Geometry: final body of the model. Coordinates: model frame, mm. Give positions to 0.01 mm unless a question says otherwise; leave off trailing zeros. Order: outer loops, then holes, each group sorted by start corner. A loop starts at its lowest first (then second) coordinate and runs counter-clockwise, first axis right, second up. Notation, with made-up numbers: M 73.25,36 L 126.25,36 A20 cw 126.25,48 Z; hole C -30.75,88.5 d4. An arc over 180 degrees is marked long. One line per item, written item: value. Start each with the question number.
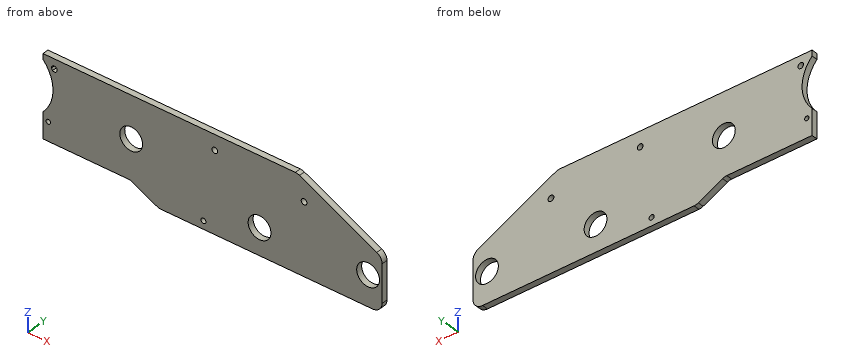
```python
from build123d import *

# Parameters (mm, degrees)
SKETCH1_W           = 210
SKETCH1_H           = 50
SKETCH1_R           = 1.211665018
SKETCH1_R_2         = 1.165617118
SKETCH1_R_3         = 1.5
SKETCH1_R_4         = 1.517273905
SKETCH1_R_5         = 1.335614121
SKETCH1_R_6         = 1.62438417
BOSS_EXTRUDE1_DEPTH = 3.175
SKETCH2_R           = 2
CUT_EXTRUDE1_DEPTH  = 10
SKETCH3_R           = 6
SKETCH3_R_2         = 0.586995366
CUT_EXTRUDE2_DEPTH  = 57.15
CUT_EXTRUDE7_DEPTH  = 10
FILLET3_R           = 5
SKETCH11_R          = 18.5
SKETCH11_R_2        = 2
BOSS_EXTRUDE4_DEPTH = 3.175
SKETCH12_R          = 21
BOSS_EXTRUDE5_DEPTH = 3.175
SKETCH13_R          = 18.85
CUT_EXTRUDE8_DEPTH  = 3.175
BOSS_EXTRUDE6_DEPTH = 3.175
FILLET4_R           = 5
SKETCH15_R          = 1.5
CUT_EXTRUDE9_DEPTH  = 10
SKETCH16_R          = 1.5
CUT_EXTRUDE10_DEPTH = 10
SKETCH17_R          = 1.5
CUT_EXTRUDE11_DEPTH = 10
CUT_EXTRUDE12_DEPTH = 10


with BuildPart() as part:
    # Sketch1 → Boss-Extrude1 (new body)
    with BuildSketch(Plane(origin=(0, 0, 0), x_dir=(1, 0, 0), z_dir=(0, 1, 0))):
        with Locations((105, -25)):
            Rectangle(SKETCH1_W, SKETCH1_H)
        with Locations(Location((3.489526233, -16.787661112, 0), (0, 0, 270))):
            Circle(SKETCH1_R, mode=Mode.SUBTRACT)
        with Locations(Location((34.37258772, -17.194005245, 0), (0, 0, 270))):
            Circle(SKETCH1_R_2, mode=Mode.SUBTRACT)
        with Locations(Location((37.520749958, -44.921198121, 0), (0, 0, 270))):
            Circle(SKETCH1_R_3, mode=Mode.SUBTRACT)
        with Locations(Location((168.975233936, -37.403209633, 0), (0, 0, 270))):
            Circle(SKETCH1_R_4, mode=Mode.SUBTRACT)
        with Locations(Location((116, -4.237214774, 0), (0, 0, 270))):
            Circle(SKETCH1_R_5, mode=Mode.SUBTRACT)
        with Locations(Location((12.257640281, -3.274812063, 0), (0, 0, 270))):
            Circle(SKETCH1_R_6, mode=Mode.SUBTRACT)
    extrude(amount=BOSS_EXTRUDE1_DEPTH)

    # Sketch2 → Cut-Extrude1 (cut)
    with BuildSketch(Plane(origin=(0, 3.175, 0), x_dir=(1, 0, 0), z_dir=(0, 1, 0))):
        with Locations(Location((10, -26, 0), (0, 0, 270))):
            Circle(SKETCH2_R)
        with Locations(Location((10, -42, 0), (0, 0, 270))):
            Circle(SKETCH2_R)
        with Locations(Location((26, -26, 0), (0, 0, 270))):
            Circle(SKETCH2_R)
        with Locations(Location((26, -42, 0), (0, 0, 270))):
            Circle(SKETCH2_R)
    extrude(amount=-CUT_EXTRUDE1_DEPTH, mode=Mode.SUBTRACT)

    # Sketch3 → Cut-Extrude2 (cut)
    with BuildSketch(Plane(origin=(0, 3.175, 0), x_dir=(1, 0, 0), z_dir=(0, 1, 0))):
        with Locations(Location((78.01026379, -28.1, 0), (0, 0, 270))):
            Circle(SKETCH3_R)
        with Locations(Location((145.531297368, -14, 0), (0, 0, 270))):
            Circle(SKETCH3_R)
        with Locations(Location((18, -34, 0), (0, 0, 270))):
            Circle(SKETCH3_R_2)
        with Locations(Location((202.646291021, -16, 0), (0, 0, 270))):
            Circle(SKETCH3_R)
    extrude(amount=-CUT_EXTRUDE2_DEPTH, mode=Mode.SUBTRACT)

    # Sketch10 → Cut-Extrude7 (cut)
    with BuildSketch(Plane(origin=(0, 3.175, 0), x_dir=(1, 0, 0), z_dir=(0, 1, 0))):
        Polygon((210, -27.859435908), (165.502877994, -50), (210, -50), align=None)
        Polygon((92.532613397, 0), (77.65477062, -7.402812063), (0, -7.402812063), (0, 0), align=None)
    extrude(amount=-CUT_EXTRUDE7_DEPTH, mode=Mode.SUBTRACT)

    # Fillet3
    fillet3_edges = [part.edges().sort_by_distance(p)[0] for p in [
        (210, 1.5875, 0),
        (0, 1.5875, 50),
        (92.532613397, 1.5875, 0),
        (210, 1.5875, 27.859435908),
        (165.502877994, 1.5875, 50),
        (77.65477062, 1.5875, 7.402812063),
        (0, 1.5875, 7.402812063),
    ]]
    fillet(fillet3_edges, radius=FILLET3_R)

    # Sketch11 → Boss-Extrude4 (add)
    with BuildSketch(Plane(origin=(0, 3.175, 0), x_dir=(1, 0, 0), z_dir=(0, 1, 0))):
        with Locations((18, -34)):
            Circle(SKETCH11_R)
        with Locations(Location((10, -26, 0), (0, 0, 270))):
            Circle(SKETCH11_R_2, mode=Mode.SUBTRACT)
        with Locations(Location((10, -42, 0), (0, 0, 270))):
            Circle(SKETCH11_R_2, mode=Mode.SUBTRACT)
        with Locations(Location((26, -26, 0), (0, 0, 270))):
            Circle(SKETCH11_R_2, mode=Mode.SUBTRACT)
        with Locations(Location((26, -42, 0), (0, 0, 270))):
            Circle(SKETCH11_R_2, mode=Mode.SUBTRACT)
    extrude(amount=-BOSS_EXTRUDE4_DEPTH)

    # Sketch12 → Boss-Extrude5 (add)
    with BuildSketch(Plane(origin=(0, 3.175, 0), x_dir=(1, 0, 0), z_dir=(0, 1, 0))):
        with Locations((18, -34)):
            Circle(SKETCH12_R)
    extrude(amount=-BOSS_EXTRUDE5_DEPTH)

    # Sketch13 → Cut-Extrude8 (cut)
    with BuildSketch(Plane(origin=(0, 3.175, 0), x_dir=(1, 0, 0), z_dir=(0, 1, 0))):
        with Locations(Location((18, -34, 0), (0, 0, 270))):
            Circle(SKETCH13_R)
    extrude(amount=-CUT_EXTRUDE8_DEPTH, mode=Mode.SUBTRACT)

    # Sketch14 → Boss-Extrude6 (add)
    with BuildSketch(Plane(origin=(0, 3.175, 0), x_dir=(1, 0, 0), z_dir=(0, 1, 0))):
        with BuildLine():
            Line((-35.83, -34.272812063), (-2.998227868, -34.272812063))
            ThreePointArc((-2.998227868, -34.272812063), (-2.272136238, -28.519079241), (0, -23.183346174))
            Line((0, -23.183346174), (0, -12.402812063))
            Line((0, -12.402812063), (0, -12.248529085))
            Line((0, -12.248529085), (0, 0.727187937))
            Line((0, 0.727187937), (-35.83, 0.727187937))
            Line((-35.83, 0.727187937), (-35.83, -34.272812063))
        make_face()
        with BuildLine():
            Line((0, 0.727187937), (0, -12.248529085))
            Line((0, -12.248529085), (0.002380891, -12.248529085))
            ThreePointArc((0.002380891, -12.248529085), (1.51944077, -8.813145304), (5, -7.402812063))
            Line((5, -7.402812063), (18, -7.402812063))
            Line((18, -7.402812063), (18, 0.727187937))
            Line((18, 0.727187937), (0, 0.727187937))
        make_face()
    extrude(amount=-BOSS_EXTRUDE6_DEPTH)

    # Fillet4
    fillet4_edges = [part.edges().sort_by_distance(p)[0] for p in [
        (-35.83, 1.5875, 34.272812063),
        (-35.83, 1.5875, -0.727187937),
        (18, 1.5875, -0.727187937),
    ]]
    fillet(fillet4_edges, radius=FILLET4_R)

    # Sketch15 → Cut-Extrude9 (cut)
    with BuildSketch(Plane(origin=(0, 3.175, 0), x_dir=(1, 0, 0), z_dir=(0, 1, 0))):
        with Locations(Location((122, -42.058139805, 0), (0, 0, 270))):
            Circle(SKETCH15_R)
    extrude(amount=-CUT_EXTRUDE9_DEPTH, mode=Mode.SUBTRACT)

    # Sketch16 → Cut-Extrude10 (cut)
    with BuildSketch(Plane(origin=(0, 3.175, 0), x_dir=(1, 0, 0), z_dir=(0, 1, 0))):
        with Locations(Location((12, -3.272812063, 0), (0, 0, 270))):
            Circle(SKETCH16_R)
    extrude(amount=-CUT_EXTRUDE10_DEPTH, mode=Mode.SUBTRACT)

    # Sketch17 → Cut-Extrude11 (cut)
    with BuildSketch(Plane(origin=(0, 3.175, 0), x_dir=(1, 0, 0), z_dir=(0, 1, 0))):
        with Locations(Location((-30.83, -15.772812063, 0), (0, 0, 270))):
            Circle(SKETCH17_R)
    extrude(amount=-CUT_EXTRUDE11_DEPTH, mode=Mode.SUBTRACT)

    # Sketch18 → Cut-Extrude12 (cut)
    with BuildSketch(Plane(origin=(0, 3.175, 0), x_dir=(1, 0, 0), z_dir=(0, 1, 0))):
        Polygon((31.601470509, -50), (31.601470509, 19.941328263), (-46.231581419, 19.941328263), (-46.231581419, -56.249580014), (31.601470509, -57.692191912), align=None)
    extrude(amount=-CUT_EXTRUDE12_DEPTH, mode=Mode.SUBTRACT)


solid = part.part
```
Q1. Section query D-D on x = 61. Return loops of the section in (y, z) (3 decimals).
Q2. Section query C-C on z = 14. Return loops of the section in (x, y) (3 decimals), and give its area (3 significant figures).
Q3. Contact query for flat-ended pins moving along their axis: pin 1 (1.8 mm diameter, centred on x = 37.52, z = 44.92, fed in from -Y); pin 2 (1.5 mm diameter, centred on x = 91, y = 2, fed in from -Z). Output: stop coordinate, or through.
Q4. Section query B-B on y = 1.05. Give the number of separate pieces and of enclosed holes in the cut face, and give its area (3 significant figures).
Q5. Ray query, line 1 along Z through (x, y) = (122, 2.5); line 2 along X through (y, z) = (2.95, 11); line 3 along X through (y, z) = (2.9, 15.5). Return the intervals inside material, ascending. Write a range as [from, to].
Q6. Section query A-A on x = 122. Return loops of the section in (y, z) (3 decimals).
Results below:
1. outline: M 0,7.403 L 3.175,7.403 L 3.175,50 L 0,50 Z
2. outline: M 31.601,0 L 139.531,0 L 139.531,3.175 L 31.601,3.175 Z; M 151.531,0 L 196.989,0 L 196.989,3.175 L 151.531,3.175 Z; M 208.303,0 L 210,0 L 210,3.175 L 208.303,3.175 Z
2. area: 492 mm2
3. pin 1: through
3. pin 2: z = 0.4
4. separate pieces: 1
4. enclosed holes: 8
4. area: 7,560 mm2
5. line 1: [0, 40.56], [43.56, 50]
5. line 2: [31.6, 140.34], [150.73, 199.33], [205.96, 210]
5. line 3: [31.6, 139.72], [151.34, 196.67], [208.63, 210]
6. outline: M 0,0 L 3.175,0 L 3.175,40.558 L 0,40.558 Z; M 0,43.558 L 3.175,43.558 L 3.175,50 L 0,50 Z
